Input: part model. Units: mm. Frame: model coordinates. A direction names the side the tool comes from. Coordinates: 2 decimals unless noted, no trailing zeros. Write each loop counter-clockwise with the first axis right and the second up, starting at its lowest first coordinate (ties: lowest second). Pieces come first, ordered by that corner, then holes.
from build123d import *

# Parameters (mm, degrees)
F1_DEPTH = 5
F3_DEPTH = 200.001


# Not quite as in the source:
# - a feature names something its author has since deleted; it is built from what else it names


with BuildPart() as f1:
    # F0 (on Right) → F1 (new body)
    with BuildSketch(Plane.YZ):
        Polygon((200, 60), (0, 60), (0, 0), (12, 50), (67.5, 50), (79.5, 0), (79.5, 50), (200, 50), align=None)
    extrude(amount=F1_DEPTH)

    # F2 (on face) → F3 (cut, through all)
    with BuildSketch(Plane.XZ):
        Polygon((2, 0), (0, 50), (0, 0), align=None)
        Polygon((5, 0), (5, 50), (3, 0), align=None)
    extrude(amount=-F3_DEPTH, mode=Mode.SUBTRACT)


solid = f1.part
Item 1: Pin query (flat end, axial travel): pin 1 Ø3 at (x, z) = (2.5, 23.5) entering from -Y; pin 2 Ø2.5 at (x, y) = (2.5, 126.5) entering from -Z; pin 3 Ø1.5 at (x, z) = (2.5, 31) entering from +Y; pin 4 Ø6 at (y, z) = (71, 31) entering from +X. Return the tip coordinate at first contact, or that it passes through.
Item 2: Access query for faces 1 (the face through (2, 139, 50)), 2 (the face through (2, 200, 55)), 3 (the face through (2.47, 72.08, 30.91)). Directions: +Z, -Z, +X, -X, +Y, -Y. A direction counts if a zero-diameter tool reaches every point of the face in a straight line with its end or side. Return the directions, or none.
Item 3: Material intervals for line 1 (Z direction, x = 3.4, y = 52.5); line 2 (Y direction, x = 3.05, z = 11); line 3 (Y direction, x = 1.55, z = 19.5), sorted ascending.
Item 4: Section query D-D, the plane y = 185. Return loops of the section in (x, z), then the cut area to 3 significant figures.
Item 5: Section query B-B, the plane x = 3.85. Return loops of the section in (y, z).
Item 6: Section query C-C, the plane z = 25. Return loops of the section in (x, y), then the cut area to 3 significant figures.
Item 7: Section query A-A, the plane z = 15. Return loops of the section in (x, y), then the cut area to 3 significant figures.
The answers:
1. pin 1: stops at y = 0
1. pin 2: stops at z = 50
1. pin 3: stops at y = 79.5
1. pin 4: stops at x = 4.36
2. face 1: -Z, +X, -X, +Y
2. face 2: +Z, -Z, +X, -X, +Y
2. face 3: -Z, +X, -X
3. line 1: z = 50 to 60
3. line 2: y = 0 to 2.64, 76.86 to 79.5
3. line 3: y = 0 to 4.68, 74.82 to 79.5
4. outline: (0, 50) - (5, 50) - (5, 60) - (0, 60) - close
4. area: 50.0 mm2
5. outline: (0, 21.25) - (5.1, 21.25) - (12, 50) - (67.5, 50) - (74.4, 21.25) - (79.5, 21.25) - (79.5, 50) - (200, 50) - (200, 60) - (0, 60) - close
6. outline: (1, 0) - (4, 0) - (4, 6) - (1, 6) - close; (1, 73.5) - (4, 73.5) - (4, 79.5) - (1, 79.5) - close
6. area: 36.0 mm2
7. outline: (1.4, 0) - (3.6, 0) - (3.6, 3.6) - (1.4, 3.6) - close; (1.4, 75.9) - (3.6, 75.9) - (3.6, 79.5) - (1.4, 79.5) - close
7. area: 15.8 mm2
